Autodesk Inventor part; units mm, degrees
ref_plane "YZ Plane" through (0, 0, 0) normal (1, 0, 0) x (0, 1, 0)
ref_plane "XZ Plane" through (0, 0, 0) normal (0, 1, 0) x (-1, 0, 0)
ref_plane "XY Plane" through (0, 0, 0) normal (0, 0, 1) x (1, 0, 0)
sketch "Sketch1" plane through (0, 0, 0) normal (0, 0, 1) x (1, 0, 0)
  line L0 (0, 0) -> (210, 0)
  line L1 (210, 0) -> (210, 110)
  line L2 (210, 110) -> (0, 110)
  line L3 (0, 110) -> (0, 0)
  line L4 (66.5, 93) -> (139.5, 93)
  line L5 (139.5, 93) -> (139.5, 67)
  line L6 (139.5, 67) -> (66.5, 67)
  line L7 (66.5, 67) -> (66.5, 93)
  line L8 (63, 0) -> (63, 50)
  line L9 (63, 50) -> (143, 50)
  line L10 (143, 50) -> (143, 0)
  line L11 (63, 50) -> (63, 110) construction
  circle A0 centre (28.854, 38) radius 15
  line L12 (139.5, 93) -> (144.5, 93)
  line L13 (144.5, 93) -> (144.5, 67)
  line L14 (144.5, 67) -> (139.5, 67)
  circle A1 centre (154.5, 90.4) radius 2.6
  circle A2 centre (154.5, 69.6) radius 2.6
  line L15 (171, 13) -> (187, 13) construction
  line L16 (171, 44) -> (187, 44) construction
  line L17 (171, 49) -> (187, 49)
  line L18 (187, 49) -> (187, 3)
  line L19 (187, 3) -> (171, 3)
  line L20 (171, 3) -> (171, 49)
  line L21 (179, 49) -> (179, 3) construction
  line L22 (63, 50) -> (61, 50)
  line L23 (61, 50) -> (61, 0)
  line L24 (143, 50) -> (145, 50)
  line L25 (145, 50) -> (145, 0)
  line L26 (63, 50) -> (63, 52)
  line L27 (143, 50) -> (143, 52)
  line L28 (143, 52) -> (63, 52)
  circle A3 centre (5, 105) radius 2
  circle A4 centre (5, 5) radius 2
  circle A5 centre (205, 5) radius 2
  circle A6 centre (205, 105) radius 2
  line L29 (5, 105) -> (0, 110) construction
  line L30 (5, 5) -> (0, 0) construction
  line L31 (205, 5) -> (210, 0) construction
  line L32 (210, 110) -> (205, 105) construction
  point P0 (103, 93)
  point P1 (105, 110)
  point P2 (66.5, 80)
  point P3 (63, 80)
  point P4 (103, 50)
  dimension "d0" = 210
  dimension "d1" = 110
  dimension "d2" = 73
  dimension "d3" = 26
  dimension "d4" = 50
  dimension "d5" = 80
  dimension "d6" = 30
  dimension "d7" = 28.854
  dimension "d8" = 38
  dimension "d9" = 63
  dimension "d11" = 5
  dimension "d12" = 5.2
  dimension "d13" = 10
  dimension "d17" = 13
  dimension "d18" = 44
  dimension "d19" = 5
  dimension "d20" = 10
  dimension "d21" = 16
  dimension "d22" = 31
  dimension "d27" = 2
  dimension "d36" = 4
  dimension "d37" = 5
  dimension "d38" = 5
extrude "Extrusion1" add sketch "Sketch1" against normal blind 5 contours L3 L2 L1 L0 L25 L24 L27 L28 L26 L22 L23 | L26 L28 L27 L9
extrude "Extrusion2" add sketch "Sketch1" against normal blind 2 contours L12 L13 L14 L5
extrude "Extrusion3" add sketch "Sketch1" against normal blind 2 contours L23 L22 L8 L0 | L10 L24 L25 L0
extrude "Extrusion4" cut sketch "Sketch1" against normal blind 2 contours L26 L28 L27 L9
fillet "Zaokrąglenie1" radius 5 4 edges at (0, 0, -2.5) (0, 110, -2.5) (210, 0, -2.5) (210, 110, -2.5)
properties part number "gora pudla"
Check sheet for the modelled part. Datum: model origin and axes. Units: mm. A direction names the side the tool comes from. Give positions to 0.01 mm unless a question says otherwise; leave off trailing zeros. Order: outer loops, then holes, each group sorted by start corner. A loop starts at its lowest first (then second) coordinate and runs counter-clockwise, first axis right, second up. Notation, with made-up numbers: M 13.25,-26 L 53.25,-26 A19 cw 53.25,-1 Z; hole C 12.5,83.25 d1. An arc over 180 degrees is marked long. Answer in a Markdown table with one row per item. Add a question column.
Q1. Sectioned sample at D-D, the plane y = 69.6. Record the boundary of the cut face in (x, z).
Q2. Thickness scan on L1, parallel to X at y = 19, z = -4.5; L2, parallel to Y at x = 205, z = -1.75; L3, parallel to Y at x = 154.5, z = -1.9. Record the ranges inside material, lowest first.
Q3. Release check for a two-part mould opening along Y. For faces 1 (the flat face through (34, 0, -2)), 2 (the flat face through (179, 49, -2)), 3 (the flat face through (210, 54, -2)), 4 (the flat face through (106, 110, -2)) record: released by +Y, released by -Y, zero draft, split by the parting line, or undercut.
Q4. Sectioned sample at A-A, the plane z = -3.9. Count the separate pieces of the cut face and the enclosed holes in it, and give its area (3 significant figures).
Q5. Access from +Z, -Z, +X, -X, +Y, -Y to the whole of each face (thin tool, end or side, straight path). Record for faces 5 (the cylindrical face through (2, 1, -3)), 6 (the flat face through (142, 80, -2)), 7 (the flat face through (171, 26, -2)).
Q6. Sectioned sample at B-B, the plane y = 38. Record the boundary of the cut face in (x, z).
Q7. Sectioned sample at C-C, the plane x = 118.5. Record the boundary of the cut face in (y, z), and give its area (3 significant figures).
Q8. Gauge pin test, flat ends, axial feed: pin 1 Ø1 at (x, y) = (143.5, 35.5) entering from -Z; pin 2 Ø1.5 at (x, z) = (103, -3) entering from -Y. Record the tip position at first contact, or that the pin passes through.
Verdict:
| question | item | result |
|---|---|---|
| 1 | outline | M 0,-5 L 66.5,-5 L 66.5,0 L 0,0 Z; M 139.5,-2 L 144.5,-2 L 144.5,-5 L 151.9,-5 L 151.9,0 L 139.5,0 Z; M 157.1,-5 L 210,-5 L 210,0 L 157.1,0 Z |
| 2 | L1 | 0 to 61, 145 to 171, 187 to 210 |
| 2 | L2 | 0 to 3, 7 to 103, 107 to 110 |
| 2 | L3 | 0 to 67, 72.2 to 87.8, 93 to 110 |
| 3 | face 1 | released by -Y |
| 3 | face 2 | undercut |
| 3 | face 3 | zero draft |
| 3 | face 4 | released by +Y |
| 4 | separate pieces | 1 |
| 4 | enclosed holes | 9 |
| 4 | area | 15,300 mm² |
| 5 | face 5 | +Z, -Z, -X, -Y |
| 5 | face 6 | -Z |
| 5 | face 7 | +Z, -Z |
| 6 | outline | M 0,-5 L 13.85,-5 L 13.85,0 L 0,0 Z; M 43.85,-5 L 61,-5 L 61,-2 L 63,-2 L 63,0 L 43.85,0 Z; M 143,-2 L 145,-2 L 145,-5 L 171,-5 L 171,0 L 143,0 Z; M 187,-5 L 210,-5 L 210,0 L 187,0 Z |
| 7 | outline | M 50,-5 L 67,-5 L 67,0 L 52,0 L 52,-2 L 50,-2 Z; M 93,-5 L 110,-5 L 110,0 L 93,0 Z |
| 7 | area | 166 mm² |
| 8 | pin 1 | z = -2 |
| 8 | pin 2 | y = 50 |
